```python
from build123d import *

# Parameters (mm, degrees)
SKETCH1_W           = 38.1
SKETCH1_H           = 76.2
BOSS_EXTRUDE1_DEPTH = 7.9375
SKETCH2_R           = 3.96875
CUT_EXTRUDE1_DEPTH  = 44.330317403
SKETCH4_R           = 9.525
CUT_EXTRUDE2_DEPTH  = 4.7625
SKETCH5_R           = 4.7625
BOSS_EXTRUDE2_DEPTH = 9.4488
SKETCH6_R           = 3.175
BOSS_EXTRUDE3_DEPTH = 6.604
SKETCH7_W           = 38.1
SKETCH7_H           = 31.75
SKETCH7_R           = 2
BOSS_EXTRUDE4_DEPTH = 7.9375


with BuildPart() as part:
    # Sketch1 → Boss-Extrude1 (new body)
    with BuildSketch(Plane.XY):
        Rectangle(SKETCH1_W, SKETCH1_H)
    extrude(amount=BOSS_EXTRUDE1_DEPTH)

    # Sketch2 → Cut-Extrude1 (cut, through all)
    with BuildSketch(Plane.XY.offset(7.9375)):
        Circle(SKETCH2_R)
    extrude(amount=-CUT_EXTRUDE1_DEPTH, mode=Mode.SUBTRACT)

    # Sketch4 → Cut-Extrude2 (cut)
    with BuildSketch(Plane.XY.offset(7.9375)):
        Circle(SKETCH4_R)
    extrude(amount=-CUT_EXTRUDE2_DEPTH, mode=Mode.SUBTRACT)

    # Sketch5 → Boss-Extrude2 (add)
    with BuildSketch(Plane.XY.offset(7.9375)):
        with Locations(Location((0, 25.4, 0), (0, 0, 180))):
            Circle(SKETCH5_R)
    boss_extrude2 = extrude(amount=BOSS_EXTRUDE2_DEPTH)

    # Sketch6 → Boss-Extrude3 (add)
    with BuildSketch(Plane.XY.offset(17.3863)):
        with Locations(Location((0, 25.4, 0), (0, 0, 180))):
            Circle(SKETCH6_R)
    boss_extrude3 = extrude(amount=BOSS_EXTRUDE3_DEPTH)

    # Mirror1: Boss-Extrude2, Boss-Extrude3 across plane
    add(boss_extrude2.mirror(Plane.ZX))
    add(boss_extrude3.mirror(Plane.ZX))

    # Sketch7 → Boss-Extrude4 (add)
    with BuildSketch(Plane.XY.offset(7.9375)):
        with Locations((0, 53.975)):
            Rectangle(SKETCH7_W, SKETCH7_H)
        with Locations((12.7, 63.5)):
            Circle(SKETCH7_R, mode=Mode.SUBTRACT)
        with Locations(Location((12.7, 44.45, 0), (0, 0, 180))):
            Circle(SKETCH7_R, mode=Mode.SUBTRACT)
    extrude(amount=-BOSS_EXTRUDE4_DEPTH)


solid = part.part
```
Can you work these out from the model? Positions are in its coordinate system, mm. A direction names the side the tool comes from. Round coordinates to 2 decimals unless told otherwise and drop trailing zeros. Order: outer loops, then holes, each group sorted by start corner. A loop starts at its lowest first (then second) coordinate and runs counter-clockwise, first axis right, second up. Notation, with made-up numbers: (-2.5, 28.5) -> (29.5, 28.5) arc R25 ccw to (29.5, 40.5) -> close; hole circle Ø7 at (81, 65). An arc over 180 degrees is marked (long way). Return JSON: item names as keys, results as strings. Group by question number.
1. We'd pull the mould along X, two halves only. Please class faces 3 (the face through (-7.559, -5.796, 5.59)), 4 (the face through (19.05, 15, 4)), 5 (the face through (0, 69.85, 4)): released by +X, released by -X, zero draft, split by the parting line, or undercut.
2. I need wall thicknesses on line 1 (Y direction, x = 0, z = 21.75) (3 decimals); line 2 (X direction, y = 44.45, z = 4.75); line 3 (Y direction, x = 11.5, z = 6.5). Which ranges of each line are inside material? Lowest first, please. Write a range as [from, to].
3. If we section it at A-A, the plane x = 12.7: Write out the boundary of the cut face in (y, z).
4. If we section it at C-C, the plane z = 6: Write out the boundary of the cut face in (x, y) (3 decimals).
5. If we section it at B-B, the plane y = 44.45: Write out the boundary of the cut face in (x, z), then the cut area to 3 significant figures.
6. Will these pins go through, and if not, where does the flat tip stop? pin 1 (3 mm diameter, centred on x = -6, z = 18.5, fed in from +Y); pin 2 (15 mm diameter, centred on x = -4.5, y = -4.5, fed in from +Z); pin 3 (4 mm diameter, centred on x = -4, z = 21.5, fed in from -Y); pin 4 (5 mm diameter, centred on x = 1.5, z = 12.5, fed in from +Y).
7. Which directions (+Z, -Z, +X, -X, +Y, -Y) give clear straight access to the entire face, cutting with the end or side of a thin tool? Please do faces 1 (the face through (-1, -29, 17.386)), 2 (the face through (0, -38.1, 4)).
Output values:
{
 "1": {"face 3": "undercut", "face 4": "released by +X", "face 5": "zero draft"},
 "2": {"line 1": "[-28.575, -22.225], [22.225, 28.575]", "line 2": "[-19.05, 10.7], [14.7, 19.05]", "line 3": "[-38.1, 42.85], [46.05, 61.9], [65.1, 69.85]"},
 "3": {"outline": "(-38.1, 0) -> (42.45, 0) -> (42.45, 7.94) -> (-38.1, 7.94) -> close; (46.45, 0) -> (61.5, 0) -> (61.5, 7.94) -> (46.45, 7.94) -> close; (65.5, 0) -> (69.85, 0) -> (69.85, 7.94) -> (65.5, 7.94) -> close"},
 "4": {"outline": "(-19.05, -38.1) -> (19.05, -38.1) -> (19.05, 69.85) -> (-19.05, 69.85) -> close; hole circle Ø19.05 at (0, 0); hole circle Ø4 at (12.7, 44.45); hole circle Ø4 at (12.7, 63.5)"},
 "5": {"outline": "(-19.05, 0) -> (10.7, 0) -> (10.7, 7.94) -> (-19.05, 7.94) -> close; (14.7, 0) -> (19.05, 0) -> (19.05, 7.94) -> (14.7, 7.94) -> close", "area": "271 mm²"},
 "6": {"pin 1": "through", "pin 2": "z = 7.94", "pin 3": "y = -27.87", "pin 4": "y = 30.16"},
 "7": {"face 1": "+Z", "face 2": "+Z, -Z, +X, -X, -Y"}
}
